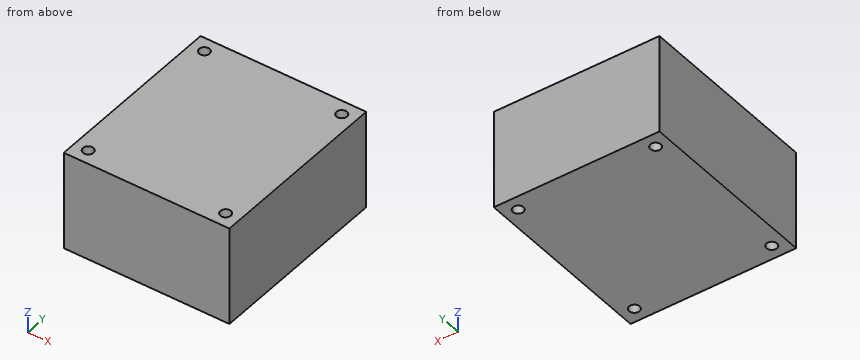
Autodesk Inventor part; units mm, degrees
ref_plane "YZ Plane" through (0, 0, 0) normal (1, 0, 0) x (0, 1, 0)
ref_plane "XZ Plane" through (0, 0, 0) normal (0, 1, 0) x (-1, 0, 0)
ref_plane "XY Plane" through (0, 0, 0) normal (0, 0, 1) x (1, 0, 0)
sketch "スケッチ1" plane through (0, 0, 0) normal (0, 0, 1) x (1, 0, 0)
  line L0 (-23.5, 26.5) -> (23.5, 26.5)
  line L1 (23.5, 26.5) -> (23.5, -26.5)
  line L2 (23.5, -26.5) -> (-23.5, -26.5)
  line L3 (-23.5, -26.5) -> (-23.5, 26.5)
  line L4 (-23.5, 26.5) -> (23.5, -26.5) construction
  line L5 (23.5, 26.5) -> (-23.5, -26.5) construction
  point P0 (0, 0)
  dimension "d0" = 47
  dimension "d1" = 53
extrude "押し出し1" add sketch "スケッチ1" along normal blind 28
sketch "スケッチ2" plane through (0, 0, 0) normal (0, 0, -1) x (-1, 0, 0)
  line L0 (23.5, -26.5) -> (23.5, 26.5)
  line L1 (23.5, -26.5) -> (-23.5, -26.5)
  line L2 (23.5, 26.5) -> (-23.5, 26.5)
  line L3 (-23.5, 26.5) -> (-23.5, -26.5)
  point P0 (0, 0)
  point P1 (19.5, -22.5)
  point P2 (19.5, 22.5)
  point P3 (-19.5, 22.5)
  point P4 (-19.5, -22.5)
  dimension "d4" = 4
  dimension "d5" = 4
  dimension "d6" = 4
  dimension "d7" = 4
hole "穴1" at (-19.5, -22.5, 0) at (-19.5, 22.5, 0) at (19.5, 22.5, 0) at (19.5, -22.5, 0) direction (0, 0, 1) diameter 3 end through all
properties part number "Motor board ver2"
The listing builds one solid part. Answer for the finished solid, in the listing's coordinates (mm). Give positions to 0.01 mm unless a question says otherwise; leave off trailing zeros. Loops run counter-clockwise (first coordinate to the right, second up) from the corner with the lowest first, then second, coordinate; pieces in that order, holes last. Notation, with made-up numbers: M 36,-13.5 L 85,-13.5 A28 ccw 85,16.5 Z; hole C 23,56.25 d1. An arc over 180 degrees is marked long. One line per item, written item: value.
Q1. Find the intervals of material crossed by line 1 (Y direction, x = -19.5, z = 7.5); line 2 (X direction, y = 22.5, z = 20.25); line 3 (Y direction, x = -20.5, z = 26), in increasing order. Write a range as from..to.
Working result:
line 1: y = -26.5..-24, -21..21, 24..26.5
line 2: x = -23.5..-21, -18..18, 21..23.5
line 3: y = -26.5..-23.62, -21.38..21.38, 23.62..26.5
Q2. A cutting plane is placed at A-A on y = 22.5. Determine the outline of the cut face in (x, z).
Working result:
outline: M -23.5,0 L -21,0 L -21,28 L -23.5,28 Z; M -18,0 L 18,0 L 18,28 L -18,28 Z; M 21,0 L 23.5,0 L 23.5,28 L 21,28 Z
Q3. A flat-ended cylindrical pin translates along its axis: P1, Ø1.8, axis at x = 19.5, y = -22.5, coming from the +Z side. Find the tip coordinate at first contact, or state that the pin passes through.
Working result:
P1: passes through
Q4. A cutting plane is placed at B-B on x = 19.5. Determine the outline of the cut face in (y, z), then the cut area to 3 significant figures.
Working result:
outline: M -26.5,0 L -24,0 L -24,28 L -26.5,28 Z; M -21,0 L 21,0 L 21,28 L -21,28 Z; M 24,0 L 26.5,0 L 26.5,28 L 24,28 Z
area: 1,320 mm^2
